Geometry: final body of the model. Coordinates: model frame, mm. Face numbers are marked on the shaded views. A direction names the side the tool comes from. Round coordinates to 2 decimals unless told otherwise and drop trailing zeros. Write each loop counter-clockwise with the first axis right and the second up, starting at its lowest first coordinate (ties: lowest second). Pieces come first, ordered by that corner, then holes. Notation, with made-up numbers: (8.25, 33.5) -> (48.25, 33.5) arc R37 cw to (48.25, 70.5) -> close; hole circle Ø2 at (9, 21). An arc over 180 degrees is marked (long way). Use one line per item in the form item = value. Start each with the question number.
1. Reachability of the marked faces 1 and 2 from +Z, -Z, +X, -X, +Y, -Y: full face, straight path, thin tool, end or side. Return the list, or none.
2. Line query: L1, parallel to Z at x = -42, y = 138.5; L2, parallel to Z at x = 72, y = 156.5; L3, parallel to X at y = 44, z = 26. Output: solid intervals per line, ascending.
3. Pin query (flat end, axial travel): pin 1 Ø3 at (x, y) = (70.5, 90) entering from +Z; pin 2 Ø5 at (x, y) = (-23.5, 56) entering from +Z; pin 3 Ø12 at (x, y) = (-101, 159.5) entering from +Z. Return the tip coordinate at first contact, or that it passes through.
4. Cut plane C-C, the plane x = -142. Return the cut outline in (y, z).
5. Cut plane A-A, the plane y = 82.5. Return the cut outline in (x, z).
6. Cut plane B-B, the plane z = 59.5. Return the cut outline in (x, y).
```python
from build123d import *

# Parameters (mm, degrees)
PAD_DEPTH = 200


with BuildPart() as part:
    # Sketch → Pad (new body)
    with BuildSketch(Plane.XZ):
        Polygon((-200, 100), (-200, 0), (0, 0), (141.421356, 141.421356), (70.710678, 212.132034), (-41.421356, 100), align=None)
    extrude(amount=-PAD_DEPTH)


solid = part.part
```
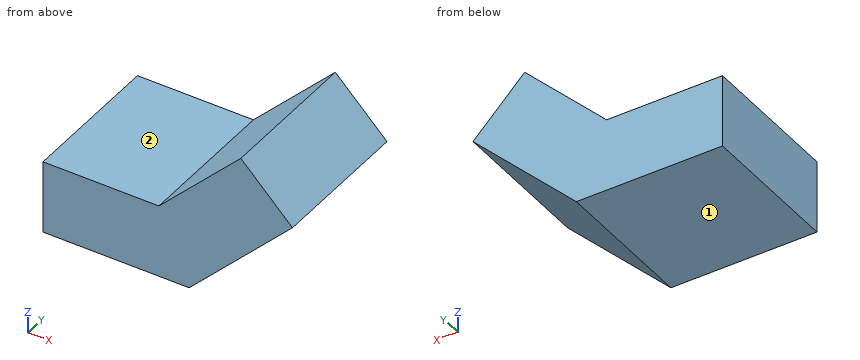
Outcome:
q1.face_1 = -Z, +X, -X, +Y, -Y
q1.face_2 = +Z, -X, +Y, -Y
q2.L1 = 0 to 100
q2.L2 = 72 to 210.84
q2.L3 = -200 to 26
q3.pin_1 = 212.13
q3.pin_2 = 120.42
q3.pin_3 = 100
q4.outline = (0, 0) -> (200, 0) -> (200, 100) -> (0, 100) -> close
q5.outline = (-200, 0) -> (0, 0) -> (141.42, 141.42) -> (70.71, 212.13) -> (-41.42, 100) -> (-200, 100) -> close
q6.outline = (-200, 0) -> (59.5, 0) -> (59.5, 200) -> (-200, 200) -> close
